For this review, take the finished solid that the model builds, in its own axes (mm). A direction names the side the tool comes from. Give positions to 0.01 mm unless a question says otherwise; leave off trailing zeros. Order: outer loops, then holes, each group sorted by start corner. A loop starts at its lowest first (then second) coordinate and runs counter-clockwise, first axis right, second up.
Item 1: For P1, Ø3, axis at x = 21, z = 0, coming from the -Y side; P2, Ø3, axis at x = 1.58, z = -4.57, coming from the -Y side, all flat-tipped, find the tip position at first contact; note any pin that passes through.
Item 2: Consider section B-B (x = -22). Give the boundary of the cut face in (y, z), plus the area to 3 significant figures.
Item 3: For probe 1 along X at (y, z) = (1, -2.75); probe 2 along X at (y, z) = (1.75, 3); probe 3 along X at (y, z) = (1.2, -5.5), list the stretches that pass through material, from the lowest coordinate up.
Item 4: The part is to be moulded in two halves that separate along Z. For faces 1 (the flat face through (1, 1, -8.319)), 2 (the flat face through (-21, 1, -6.319)), 3 (the flat face through (28.626, 1, -1)), say which applies: released by +Z, released by -Z, zero draft, split by the parting line, or undercut.
Item 5: Consider section C-C (y = 1.2). Give the boundary of the cut face in (x, z), plus the area to 3 significant figures.
Item 6: Machinability: for faces 4 (the flat face through (1, 0, -1)), 5 (the flat face through (-23.474, 1, -1)), which of the approach directions +Z, -Z, +X, -X, +Y, -Y give a long, thin tool a straight path to every point of the face, cutting with its end or side? Answer none if there is none.
Item 7: Consider section D-D (z = 2.25). Give the boundary of the cut face in (x, y).
Item 8: Consider section A-A (z = -1). Give the boundary of the cut face in (x, y).
```python
from build123d import *

# Parameters (mm, degrees)
SKETCH1_W           = 54.1
SKETCH1_H           = 15
SKETCH1_R           = 1.75
SKETCH1_W_2         = 6
SKETCH1_H_2         = 11
BOSS_EXTRUDE1_DEPTH = 2


with BuildPart() as part:
    # Sketch1 → Boss-Extrude1 (new body)
    with BuildSketch(Plane(origin=(0, 0, 0), x_dir=(1, 0, 0), z_dir=(0, 1, 0))):
        with Locations((1.576423546, 0.819405027)):
            Rectangle(SKETCH1_W, SKETCH1_H)
        with Locations(Location((16.756423546, -3.190594973, 0), (0, 0, 270))):
            Circle(SKETCH1_R, mode=Mode.SUBTRACT)
        with Locations(Location((-13.603576454, -3.190594973, 0), (0, 0, 270))):
            Circle(SKETCH1_R, mode=Mode.SUBTRACT)
        with Locations(Location((1.576423546, 4.569405027, 0), (0, 0, 270))):
            Circle(SKETCH1_R, mode=Mode.SUBTRACT)
        with Locations((-20.473576454, 0.819405027)):
            Rectangle(SKETCH1_W_2, SKETCH1_H_2, mode=Mode.SUBTRACT)
        with Locations((23.626423546, 0.819405027)):
            Rectangle(SKETCH1_W_2, SKETCH1_H_2, mode=Mode.SUBTRACT)
    extrude(amount=BOSS_EXTRUDE1_DEPTH)


solid = part.part
```
Resolved:
1. P1: stops at y = 0
1. P2: passes through
2. outline: (0, -8.32) - (2, -8.32) - (2, -6.32) - (0, -6.32) - close; (0, 4.68) - (2, 4.68) - (2, 6.68) - (0, 6.68) - close
2. area: 8.00 mm2
3. probe 1: x = -25.47 to -23.47, -17.47 to 20.63, 26.63 to 28.63
3. probe 2: x = -25.47 to -23.47, -17.47 to -15.34, -11.86 to 15.02, 18.5 to 20.63, 26.63 to 28.63
3. probe 3: x = -25.47 to -23.47, -17.47 to 0.09, 3.06 to 20.63, 26.63 to 28.63
4. face 1: released by -Z
4. face 2: undercut
4. face 3: zero draft
5. outline: (-25.47, -8.32) - (28.63, -8.32) - (28.63, 6.68) - (-25.47, 6.68) - close; hole (-23.47, -6.32) - (-17.47, -6.32) - (-17.47, 4.68) - (-23.47, 4.68) - close; hole circle Ø3.5 at (-13.6, 3.19); hole circle Ø3.5 at (1.58, -4.57); hole circle Ø3.5 at (16.76, 3.19); hole (20.63, -6.32) - (26.63, -6.32) - (26.63, 4.68) - (20.63, 4.68) - close
5. area: 651 mm2
6. face 4: +Z, -Z, +X, -X, -Y
6. face 5: +Y, -Y
7. outline: (-25.47, 0) - (-23.47, 0) - (-23.47, 2) - (-25.47, 2) - close; (-17.47, 0) - (-15.08, 0) - (-15.08, 2) - (-17.47, 2) - close; (-12.13, 0) - (15.28, 0) - (15.28, 2) - (-12.13, 2) - close; (18.23, 0) - (20.63, 0) - (20.63, 2) - (18.23, 2) - close; (26.63, 0) - (28.63, 0) - (28.63, 2) - (26.63, 2) - close
8. outline: (-25.47, 0) - (-23.47, 0) - (-23.47, 2) - (-25.47, 2) - close; (-17.47, 0) - (20.63, 0) - (20.63, 2) - (-17.47, 2) - close; (26.63, 0) - (28.63, 0) - (28.63, 2) - (26.63, 2) - close
